```python
from build123d import *

# Parameters (mm, degrees)
SKETCH1_W           = 105.949999994
SKETCH1_H           = 98.843650928
BOSS_EXTRUDE1_DEPTH = 19.05
SKETCH2_R           = 30.7975
CUT_EXTRUDE1_DEPTH  = 499.69403033
CHAMFER1_SIZE       = 6.35


with BuildPart() as part:
    # Sketch1 → Boss-Extrude1 (new body)
    with BuildSketch(Plane.XY):
        with Locations((0, 446.084463863)):
            Rectangle(SKETCH1_W, SKETCH1_H)
    extrude(amount=-BOSS_EXTRUDE1_DEPTH)

    # Sketch2 → Cut-Extrude1 (cut, through all)
    with BuildSketch(Plane.XY):
        with Locations((0, 457.406289235)):
            Circle(SKETCH2_R)
    extrude(amount=-CUT_EXTRUDE1_DEPTH, mode=Mode.SUBTRACT)

    # Chamfer1
    chamfer1_edges = [part.edges().sort_by_distance(p)[0] for p in [
        (52.974999997, 396.662638399, -9.525),
        (-52.974999997, 396.662638399, -9.525),
    ]]
    chamfer(chamfer1_edges, length=CHAMFER1_SIZE)


solid = part.part
```
Model file for the job. Use its own axes, mm. Give positions to 0.01 mm unless a question says otherwise; leave off trailing zeros. Write each loop counter-clockwise with the first axis right and the second up, starting at its lowest first coordinate (ties: lowest second). Pieces come first, ordered by that corner, then holes. Notation, with made-up numbers: (82.5, 14.5) -> (114.5, 14.5) arc R30 cw to (114.5, 38.5) -> close; hole circle Ø5 at (40, 3.5). An arc over 180 degrees is marked (long way). Use CSV: the item, a comma, the result in double quotes. Start each with the question number.
1) Drill centre lines: L1, parallel to Y at x = 0, z = -9.5; L2, parallel to X at y = 432, z = -5 (3 decimals); L3, parallel to X at y = 484, z = -7.75 (3 decimals). Where is each one in solid material? Low to high.
2) Cut at C-C on z = -16.75. List the corners of the cut face in (x, y) (1 decimal).
3) Cut at A-A on x = 0. List the corners of the cut face in (y, z).
4) Cut at B-B on y = 437.5. List the corners of the cut face in (x, z) (3 decimals), plus the area to 3 significant figures.
5) Two-plate mould, pull along Y, no slides. Class faces 1 (the cylindrical face through (14.211, 430.084, -9.392)), 2 (the flat face through (49.84, 399.88, -9.39)), 3 (the flat face through (-1, 495.506, -9)), 4 (the flat face through (52.975, 449, -9)): released by +Y, released by -Y, zero draft, split by the parting line, or undercut.
Final values:
1,L1,"y = 396.66 to 426.61, 488.2 to 495.51"
1,L2,"x = -52.975 to -17.407, 17.407 to 52.975"
1,L3,"x = -52.975 to -15.533, 15.533 to 52.975"
2,outline,"(-53, 403) -> (-46.6, 396.7) -> (46.6, 396.7) -> (53, 403) -> (53, 495.5) -> (-53, 495.5) -> close; hole circle Ø61.6 at (0, 457.4)"
3,outline,"(396.66, -19.05) -> (426.61, -19.05) -> (426.61, 0) -> (396.66, 0) -> close; (488.2, -19.05) -> (495.51, -19.05) -> (495.51, 0) -> (488.2, 0) -> close"
4,outline,"(-52.975, -19.05) -> (-23.499, -19.05) -> (-23.499, 0) -> (-52.975, 0) -> close; (23.499, -19.05) -> (52.975, -19.05) -> (52.975, 0) -> (23.499, 0) -> close"
4,area,"1,120 mm2"
5,face 1,"undercut"
5,face 2,"released by -Y"
5,face 3,"released by +Y"
5,face 4,"zero draft"
